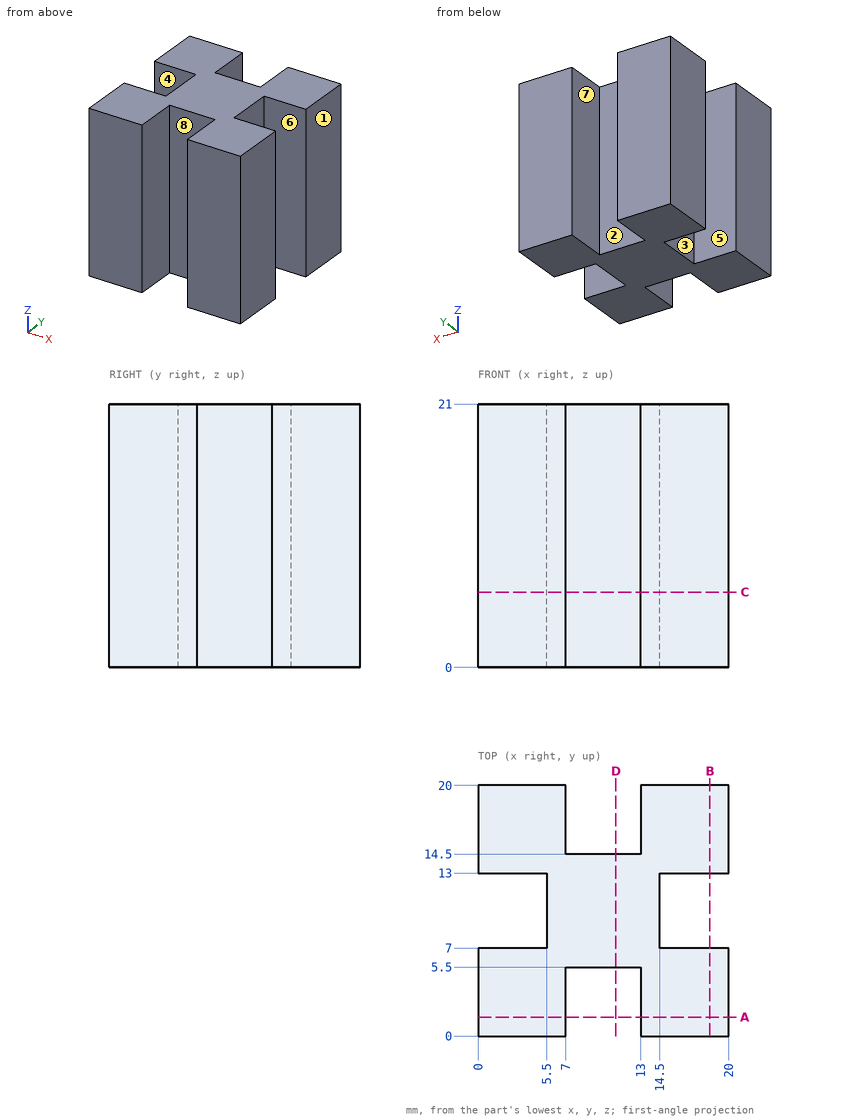
The drawing under review shows one solid part. Ordinate dimensions are in mm from its lowest x, y, z. A direction names the side the tool comes from. Round coordinates to 2 decimals unless told otherwise and drop trailing zeros. Order: outer loops, then holes, each group sorted by start corner. A loop starts at its lowest first (then second) coordinate and runs counter-clockwise, first axis right, second up. Notation, with made-up numbers: (81.25, 26.25) - (97.25, 26.25) arc R30 cw to (97.25, 50.25) - close; hole circle Ø8 at (-20.75, 79). An arc over 180 degrees is marked (long way). Return JSON: item names as keys, results as strings.
Q1. Consider section D-D on x = 11. Write out the cut boundary in (y, z).
Computed values:
{"outline": "(5.5, 0) - (14.5, 0) - (14.5, 21) - (5.5, 21) - close"}
Q2. Consider section A-A on y = 1.5. Write out the cut boundary in (x, z), plus the area to 3 significant figures.
Computed values:
{"outline": "(0, 0) - (7, 0) - (7, 21) - (0, 21) - close; (13, 0) - (20, 0) - (20, 21) - (13, 21) - close", "area": "294 mm2"}
Q3. For pin 1 Ø3 at (x, z) = (10.5, 12) entering from -Y; pin 2 Ø1.8 at (y, z) = (9.5, 8.5) entering from +X; pin 3 Ø3 at (x, z) = (9.5, 10) entering from +Y, all flat-tipped, find the tip position at first contact; note any pin that passes through.
Computed values:
{"pin 1": "stops at y = 5.5", "pin 2": "stops at x = 14.5", "pin 3": "stops at y = 14.5"}
Q4. Machinability: for the marked faces 5, 6, 7 and 8, which of the approach directions +Z, -Z, +X, -X, +Y, -Y give a long, thin tool a straight path to every point of the face, cutting with its end or side? Answer none if there is none.
Computed values:
{"face 5": "+Z, -Z, -X", "face 6": "+Z, -Z, +X", "face 7": "+Z, -Z, +Y", "face 8": "+Z, -Z, -Y"}
Q5. Wall thickness on L1, parallel to X at y = 17.5, z = 9.25; L2, parallel to X at y = 7.25, z = 10.5: over which ranges is each line inside the solid? List them lowest first. Write a range as [from, to].
Computed values:
{"L1": "x = [0, 7], [13, 20]", "L2": "x = [5.5, 14.5]"}
Q6. Consider section C-C on z = 6. Write out the cut boundary in (x, y), plus the area to 3 significant figures.
Computed values:
{"outline": "(0, 0) - (7, 0) - (7, 5.5) - (13, 5.5) - (13, 0) - (20, 0) - (20, 7) - (14.5, 7) - (14.5, 13) - (20, 13) - (20, 20) - (13, 20) - (13, 14.5) - (7, 14.5) - (7, 20) - (0, 20) - (0, 13) - (5.5, 13) - (5.5, 7) - (0, 7) - close", "area": "268 mm2"}
Q7. The part is to be moulded in two halves that separate along X. For the marked faces 1, 2, 3 and 4, say which applies: pulls with the +X half, pulls with the -X half, needs draft (parallel to the pull), parting line crosses it, or undercut.
Computed values:
{"face 1": "pulls with the +X half", "face 2": "undercut", "face 3": "pulls with the -X half", "face 4": "needs draft"}
